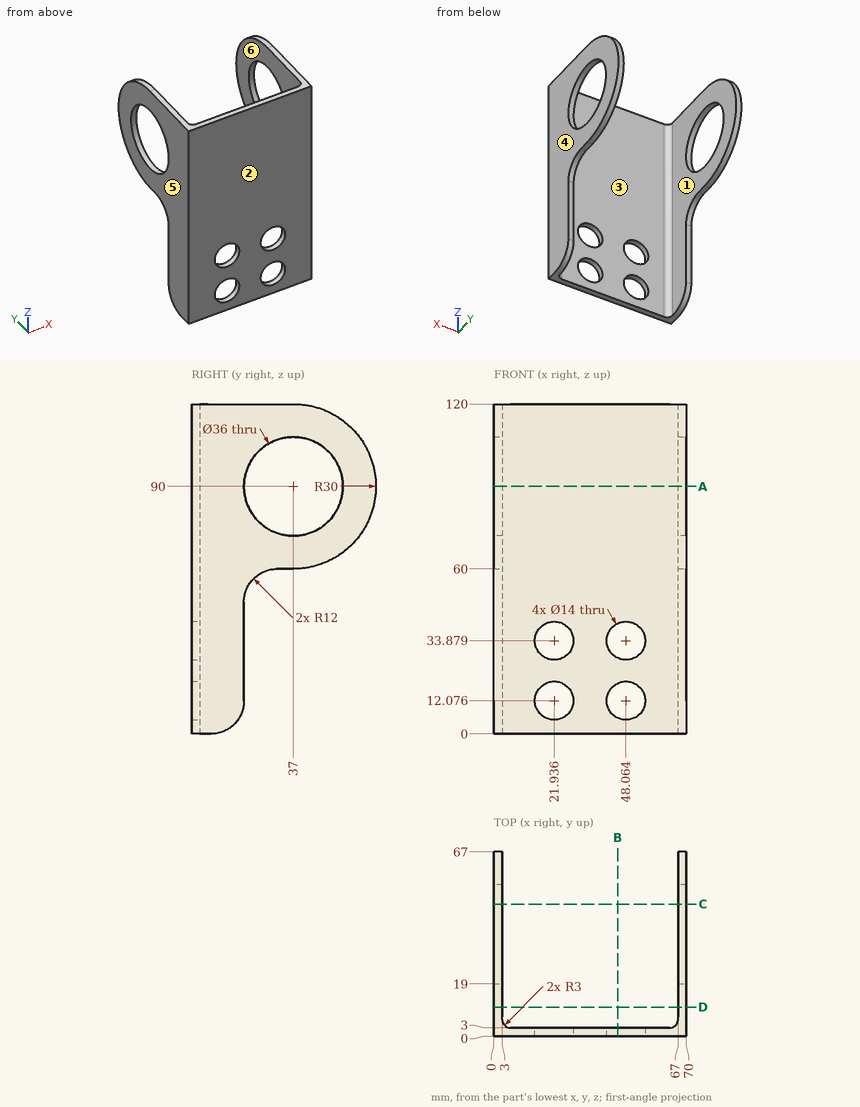
Answer from the drawing. Dimensions are ordinates in mm from the lowest x, y and z of the part. A direction names the side the tool comes from. Coordinates: 2 decimals unless noted, no trailing zeros. Write each loop counter-clockwise with the first axis right and the second up, starting at its lowest first coordinate (ties: lowest second). Pieces come first, ordered by that corner, then holes. Notation, with made-up numbers: (-24.75, 37.5) - (11.25, 37.5) arc R16 cw to (11.25, 63.5) - close; hole circle Ø9 at (53.5, 44). An arc over 180 degrees is marked (long way). Return JSON: item names as keys, results as strings. Group by question number.
Q1. Flat-ended cylindrical pins translate along their axes: pin 1 Ø3.5 at (x, y) = (1, 35.5) entering from -Z; pin 2 Ø5 at (x, z) = (27.5, 50.5) entering from +Y; pin 3 Ø1.5 at (x, z) = (69, 23.5) entering from +Y. Find the tip coordinate at first contact, or state that the pin passes through.
Q2. The part is cut by section D-D on y = 10.5. Write down the section's boundary in (x, z), and give its area (3 significant figures).
Q3. For a pull along X with two mould halves and no side action, classify the marked faces 3, 4, 5 and 6 as +X half, -X half, draft (parallel to the pull), parting line (faces both ways), or undercut.
Q4. Which of the six approach directions +Z, -Z, +X, -X, +Y, -Y give full straight-line access (tool end or side, diameter ignored) to the marked faces 1 and 2?
Q5. The part is cut by section B-B on x = 45. Write down the section's boundary in (y, z) (1 decimal).
Q6. The part is cut by section A-A on z = 90. Write down the section's boundary in (x, y), and give its area (3 significant figures).
Q7. The part is cut by section C-C on y = 48. Write down the section's boundary in (x, z), and give its area (3 significant figures).
Q8. Find the intervals of material crossed by line 1 along X through (y, z) = (15, 58); line 2 along Y through (x, z) = (2.2, 90); line 3 along Z through (x, y) = (68.7, 37), in increasing order. Write a range as [from, to].
Evaluation:
{
 "1": {"pin 1": "stops at z = 60", "pin 2": "stops at y = 3", "pin 3": "stops at y = 19"},
 "2": {"outline": "(0, 0.52) - (3, 0.52) - (3, 120) - (0, 120) - close; (67, 0.52) - (70, 0.52) - (70, 120) - (67, 120) - close", "area": "717 mm2"},
 "3": {"face 3": "undercut", "face 4": "+X half", "face 5": "-X half", "face 6": "undercut"},
 "4": {"face 1": "+Z, -Z, +Y", "face 2": "+Z, -Z, +X, -X, -Y"},
 "5": {"outline": "(0, 0) - (3, 0) - (3, 5.8) - (0, 5.8) - close; (0, 18.4) - (3, 18.4) - (3, 27.6) - (0, 27.6) - close; (0, 40.2) - (3, 40.2) - (3, 120) - (0, 120) - close"},
 "6": {"outline": "(0, 0) - (70, 0) - (70, 19) - (67, 19) - (67, 6) arc R3 cw to (64, 3) - (6, 3) arc R3 cw to (3, 6) - (3, 19) - (0, 19) - close; (0, 55) - (3, 55) - (3, 67) - (0, 67) - close; (67, 55) - (70, 55) - (70, 67) - (67, 67) - close", "area": "382 mm2"},
 "7": {"outline": "(0, 62.09) - (3, 62.09) - (3, 75.75) - (0, 75.75) - close; (0, 104.25) - (3, 104.25) - (3, 117.91) - (0, 117.91) - close; (67, 62.09) - (70, 62.09) - (70, 75.75) - (67, 75.75) - close; (67, 104.25) - (70, 104.25) - (70, 117.91) - (67, 117.91) - close", "area": "164 mm2"},
 "8": {"line 1": "x = [0, 3], [67, 70]", "line 2": "y = [0, 19], [55, 67]", "line 3": "z = [60, 72], [108, 120]"}
}
